Input: part model. Units: mm. Frame: model coordinates. Face numbers are marked on the shaded views. A direction names the side the tool comes from. Round coordinates to 2 decimals unless told otherwise and drop trailing zeros. Order: outer loops, then holes, each group sorted by start corner. A loop starts at its lowest first (then second) coordinate and runs counter-clockwise, first axis right, second up. Notation, with made-up numbers: (25.25, 11) - (82.25, 11) arc R17 ccw to (82.25, 40) - close; hole circle Ø7 at (47, -31.5). An arc over 180 degrees is marked (long way). One line per item, written item: value. Start each with the question number.
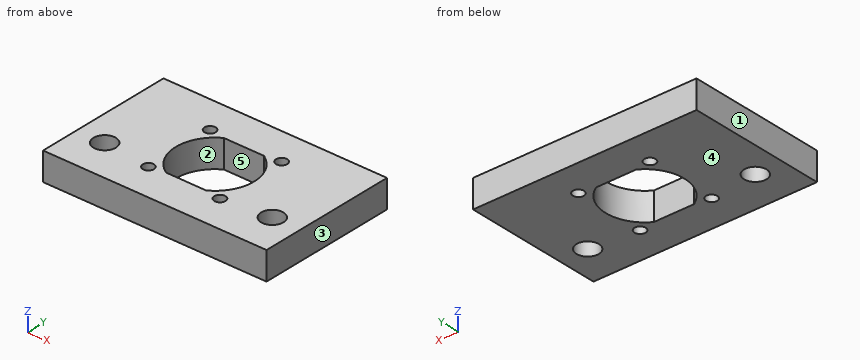
from build123d import *

# Parameters (mm, degrees)
SKETCH1_W           = 40
SKETCH1_H           = 25
SKETCH1_R           = 2
SKETCH1_R_2         = 1
BOSS_EXTRUDE1_DEPTH = 5


with BuildPart() as part:
    # Sketch1 → Boss-Extrude1 (new body)
    with BuildSketch(Plane.XY):
        Rectangle(SKETCH1_W, SKETCH1_H)
        with Locations((15, -5.5)):
            Circle(SKETCH1_R, mode=Mode.SUBTRACT)
        with Locations((-6.4, 6.4)):
            Circle(SKETCH1_R_2, mode=Mode.SUBTRACT)
        with Locations((-15, -5.5)):
            Circle(SKETCH1_R, mode=Mode.SUBTRACT)
        with Locations((6.4, 6.4)):
            Circle(SKETCH1_R_2, mode=Mode.SUBTRACT)
        with Locations((6.4, -6.4)):
            Circle(SKETCH1_R_2, mode=Mode.SUBTRACT)
        with Locations((-6.4, -6.4)):
            Circle(SKETCH1_R_2, mode=Mode.SUBTRACT)
        with BuildLine():
            Line((-3.605551275, 6), (3.605551275, 6))
            ThreePointArc((3.605551275, 6), (7, 0), (3.605551275, -6))
            Line((3.605551275, -6), (-3.605551275, -6))
            ThreePointArc((-3.605551275, -6), (-7, 0), (-3.605551275, 6))
        make_face(mode=Mode.SUBTRACT)
    extrude(amount=BOSS_EXTRUDE1_DEPTH)


solid = part.part
1. Section D-D (y = 3.5). Return the cut outline in (x, z).
2. Line query: line 1 (Y direction, x = 2.5, z = 1.9); line 2 (X direction, y = 0.25, z = 1.45); line 3 (Y direction, x = 15, z = 2.05). Output: solid intervals per line, ascending. Write a range as from..to.
3. Set-up query: the marked faces 1 and 2. Return all of +Z, -Z, +X, -X, +Y, -Y with unobstructed straight access to the full face (end or side cutting, diameter ignored); none if empty.
4. Section B-B (x = 15). Return the cut outline in (y, z).
5. Section A-A (z = 2.55). Return the cut outline in (x, y).
6. Pull-direction query (X, two-part tool) for the marked faces 3, 4 and 5; classes: released by +X, released by -X, zero draft, split by the parting line, or undercut.
7. Section C-C (y = 6.4). Return the cut outline in (x, z).
8. Pin query (flat end, axial travel): pin 1 (1.6 mm diameter, centred on x = -6.4, y = -6.4, fed in from +Z). Return the tip coordinate at first contact, or that it passes through.
Solved:
1. outline: (-20, 0) - (-6.06, 0) - (-6.06, 5) - (-20, 5) - close; (6.06, 0) - (20, 0) - (20, 5) - (6.06, 5) - close
2. line 1: y = -12.5..-6, 6..12.5
2. line 2: x = -20..-7, 7..20
2. line 3: y = -12.5..-7.5, -3.5..12.5
3. face 1: +Z, -Z, -X, +Y, -Y
3. face 2: +Z, -Z
4. outline: (-12.5, 0) - (-7.5, 0) - (-7.5, 5) - (-12.5, 5) - close; (-3.5, 0) - (12.5, 0) - (12.5, 5) - (-3.5, 5) - close
5. outline: (-20, -12.5) - (20, -12.5) - (20, 12.5) - (-20, 12.5) - close; hole circle Ø4 at (-15, -5.5); hole circle Ø2 at (-6.4, -6.4); hole circle Ø2 at (-6.4, 6.4); hole (-3.61, -6) - (3.61, -6) arc R7 ccw to (3.61, 6) - (-3.61, 6) arc R7 ccw to start; hole circle Ø2 at (6.4, -6.4); hole circle Ø2 at (6.4, 6.4); hole circle Ø4 at (15, -5.5)
6. face 3: released by +X
6. face 4: zero draft
6. face 5: undercut
7. outline: (-20, 0) - (-7.4, 0) - (-7.4, 5) - (-20, 5) - close; (-5.4, 0) - (5.4, 0) - (5.4, 5) - (-5.4, 5) - close; (7.4, 0) - (20, 0) - (20, 5) - (7.4, 5) - close
8. pin 1: passes through
